```python
from build123d import *

# Parameters (mm, degrees)
SKETCH1_W           = 66.137036943
SKETCH1_H           = 27.94
SKETCH1_R           = 1.4
SKETCH1_R_2         = 1.45
SKETCH1_R_3         = 1.5
SKETCH1_R_4         = 1.55
SKETCH1_R_5         = 1.6
SKETCH1_R_6         = 2.5
SKETCH1_R_7         = 2.55
SKETCH1_R_8         = 2.6
SKETCH1_R_9         = 2.65
SKETCH1_R_10        = 2.7
SKETCH1_R_11        = 2.75
SKETCH1_W_2         = 2.54
SKETCH1_H_2         = 7.62
SKETCH1_H_3         = 2.54
BOSS_EXTRUDE1_DEPTH = 8.89
SKETCH2_W           = 33.530167106
SKETCH2_H           = 3.206730365
CUT_EXTRUDE1_DEPTH  = 9.89


with BuildPart() as part:
    # Sketch1 → Boss-Extrude1 (new body)
    with BuildSketch(Plane(origin=(0, 0, 0), x_dir=(1, 0, 0), z_dir=(0, 1, 0))):
        with Locations((33.068518471, 13.97)):
            Rectangle(SKETCH1_W, SKETCH1_H)
        with Locations((15.24, 20.32)):
            Circle(SKETCH1_R, mode=Mode.SUBTRACT)
        with Locations((21.59, 20.32)):
            Circle(SKETCH1_R_2, mode=Mode.SUBTRACT)
        with Locations((27.94, 20.32)):
            Circle(SKETCH1_R_3, mode=Mode.SUBTRACT)
        with Locations((34.29, 20.32)):
            Circle(SKETCH1_R_4, mode=Mode.SUBTRACT)
        with Locations((40.64, 20.32)):
            Circle(SKETCH1_R_5, mode=Mode.SUBTRACT)
        with Locations((16.51, 7.62)):
            Circle(SKETCH1_R_6, mode=Mode.SUBTRACT)
        with Locations((25.4, 7.62)):
            Circle(SKETCH1_R_7, mode=Mode.SUBTRACT)
        with Locations((34.29, 7.62)):
            Circle(SKETCH1_R_8, mode=Mode.SUBTRACT)
        with Locations((43.18, 7.62)):
            Circle(SKETCH1_R_9, mode=Mode.SUBTRACT)
        with Locations((52.07, 7.62)):
            Circle(SKETCH1_R_10, mode=Mode.SUBTRACT)
        with Locations((60.96, 7.62)):
            Circle(SKETCH1_R_11, mode=Mode.SUBTRACT)
        with Locations((3.81, 20.32)):
            Rectangle(SKETCH1_W_2, SKETCH1_H_2, mode=Mode.SUBTRACT)
        with Locations((8.89, 20.32)):
            Rectangle(SKETCH1_W_2, SKETCH1_H_2, mode=Mode.SUBTRACT)
        with Locations((3.81, 10.16)):
            Rectangle(SKETCH1_W_2, SKETCH1_H_3, mode=Mode.SUBTRACT)
        with Locations((8.89, 10.16)):
            Rectangle(SKETCH1_W_2, SKETCH1_H_3, mode=Mode.SUBTRACT)
        with Locations((3.81, 5.08)):
            Rectangle(SKETCH1_W_2, SKETCH1_H_3, mode=Mode.SUBTRACT)
        with Locations((8.89, 5.08)):
            Rectangle(SKETCH1_W_2, SKETCH1_H_3, mode=Mode.SUBTRACT)
    extrude(amount=BOSS_EXTRUDE1_DEPTH)

    # Sketch2 → Cut-Extrude1 (cut, through all)
    with BuildSketch(Plane(origin=(0, 8.89, 0), x_dir=(1, 0, 0), z_dir=(0, 1, 0))):
        with Locations((29.845478727, 26.336634818)):
            Rectangle(SKETCH2_W, SKETCH2_H)
        Polygon((66.137036943, 27.94), (46.61056228, 27.94), (46.61056228, 24.733269635), (46.61056228, 14.65880598), (66.137036943, 14.65880598), align=None)
    extrude(amount=-CUT_EXTRUDE1_DEPTH, mode=Mode.SUBTRACT)


solid = part.part
```
The listing builds one solid part. Answer for the finished solid, in the listing's coordinates (mm). A direction names the side the tool comes from. Round coordinates to 2 decimals unless told otherwise and drop trailing zeros. Order: outer loops, then holes, each group sorted by start corner. A loop starts at its lowest first (then second) coordinate and runs counter-clockwise, first axis right, second up. Notation, with made-up numbers: (-1.5, 10) -> (5.5, 10) arc R11 ccw to (5.5, 16) -> close; hole circle Ø4 at (38.25, -33.75). An arc over 180 degrees is marked (long way). Answer as CSV lines item,"result". Start each with the question number.
(1) Find the intervals of material crossed by probe 1 along Z at (x, y) = (34.29, 2.5); probe 2 along X at (y, z) = (6.25, -18.5); probe 3 along Z at (x, y) = (8.5, 1.25), in increasing order. Write a range as from..to.
(2) The part is cut by section C-C (x = 34.29). Determine the outline of the cut face in (y, z).
(3) For a pull along Z with two mould halves and no side action, classify faces 3 (the face through (10.16, 4, -5)), 4 (the face through (0, 4, -14)), 5 (the face through (10.16, 4, -20)) as +Z half, -Z half, draft (parallel to the pull), parting line (faces both ways), or undercut.
(4) The part is cut by section A-A (x = 60.96). Determine the outline of the cut face in (y, z).
(5) The part is cut by section B-B (z = -7.62). Determine the outline of the cut face in (x, y).
(6) The part is cut by section D-D (x = 52.07). Determine the outline of the cut face in (y, z).
(7) Flat-ended cylindrical pins translate along their axes: pin 1 Ø1.5 at (x, y) = (48.5, 6) entering from -Z; pin 2 Ø5 at (x, y) = (48.5, 5) entering from -Z; pin 3 Ø4 at (y, z) = (6.5, -22) entering from +X. Find the tip coordinate at first contact, or state that the pin passes through.
(8) A tool of negligible diameter and unlimited length cuts with its end or side. For faces 1 (the face through (5.08, 4, -20)), 2 (the face through (33, 8.89, -11)), from which of +Z, -Z, +X, -X, +Y, -Y can it reach the whole face along a straight path? Write none if from no direction.
Evaluation:
1,probe 1,"-24.73..-21.87, -18.77..-10.22, -5.02..0"
1,probe 2,"0..2.54, 5.08..7.62, 10.16..46.61"
1,probe 3,"-27.94..-24.13, -16.51..-11.43, -8.89..-6.35, -3.81..0"
2,outline,"(0, -24.73) -> (8.89, -24.73) -> (8.89, -21.87) -> (0, -21.87) -> close; (0, -18.77) -> (8.89, -18.77) -> (8.89, -10.22) -> (0, -10.22) -> close; (0, -5.02) -> (8.89, -5.02) -> (8.89, 0) -> (0, 0) -> close"
3,face 3,"undercut"
3,face 4,"draft"
3,face 5,"undercut"
4,outline,"(0, -14.66) -> (8.89, -14.66) -> (8.89, -10.37) -> (0, -10.37) -> close; (0, -4.87) -> (8.89, -4.87) -> (8.89, 0) -> (0, 0) -> close"
5,outline,"(0, 0) -> (14.01, 0) -> (14.01, 8.89) -> (0, 8.89) -> close; (19.01, 0) -> (22.85, 0) -> (22.85, 8.89) -> (19.01, 8.89) -> close; (27.95, 0) -> (31.69, 0) -> (31.69, 8.89) -> (27.95, 8.89) -> close; (36.89, 0) -> (40.53, 0) -> (40.53, 8.89) -> (36.89, 8.89) -> close; (45.83, 0) -> (49.37, 0) -> (49.37, 8.89) -> (45.83, 8.89) -> close; (54.77, 0) -> (58.21, 0) -> (58.21, 8.89) -> (54.77, 8.89) -> close; (63.71, 0) -> (66.14, 0) -> (66.14, 8.89) -> (63.71, 8.89) -> close"
6,outline,"(0, -14.66) -> (8.89, -14.66) -> (8.89, -10.32) -> (0, -10.32) -> close; (0, -4.92) -> (8.89, -4.92) -> (8.89, 0) -> (0, 0) -> close"
7,pin 1,"z = -14.66"
7,pin 2,"z = -24.73"
7,pin 3,"x = 46.61"
8,face 1,"+Y, -Y"
8,face 2,"+Z, -Z, +X, -X, +Y"
